Input: dimensioned drawing with shaded views. Units: mm. Origin: part minimum x, y, z. Coordinates: 2 decimals unless noted, no trailing zeros. Order: outer loops, then holes, each group sorted by start corner. A loop starts at its lowest first (then second) coordinate and runs counter-clockwise, first axis right, second up. Notation, with made-up numbers: (-30, 5) - (-18, 5) arc R25 cw to (-18, 41) - close; hole circle Ø9 at (78.5, 4.25). An arc over 180 degrees is marked (long way). Answer as CSV lines item,"result". Start each with the question number.
Item 1: Material intervals for line 1 along X through (y, z) = (8.5, 15.5); line 2 along X through (y, z) = (4.25, 13.5); line 3 along Z through (x, y) = (123.5, 12.75), sorted ascending.
Item 2: Draft query along X for the marked faces 1, 2 and 3. Return one class per face: +X half, -X half, draft (parallel to the pull), parting line (faces both ways), or undercut.
Item 3: Section A-A (y = 4.75). Output: boundary loops of the cut face in (x, z).
Item 4: Section C-C (z = 144.5). Output: boundary loops of the cut face in (x, y), and give its area (3 significant figures).
Item 5: First-contact query: pin 1 (2 mm diameter, centred on y = 3.5, z = 140, fed in from -X); pin 2 (8 mm diameter, centred on y = 6.5, z = 134.5, fed in from -X); pin 3 (8 mm diameter, centred on x = 103, y = 12.5, fed in from +Z). Flat tips, straight axial feed; report the tip coordinate or a pass-through.
Item 6: Section B-B (x = 76.2). Output: boundary loops of the cut face in (y, z).
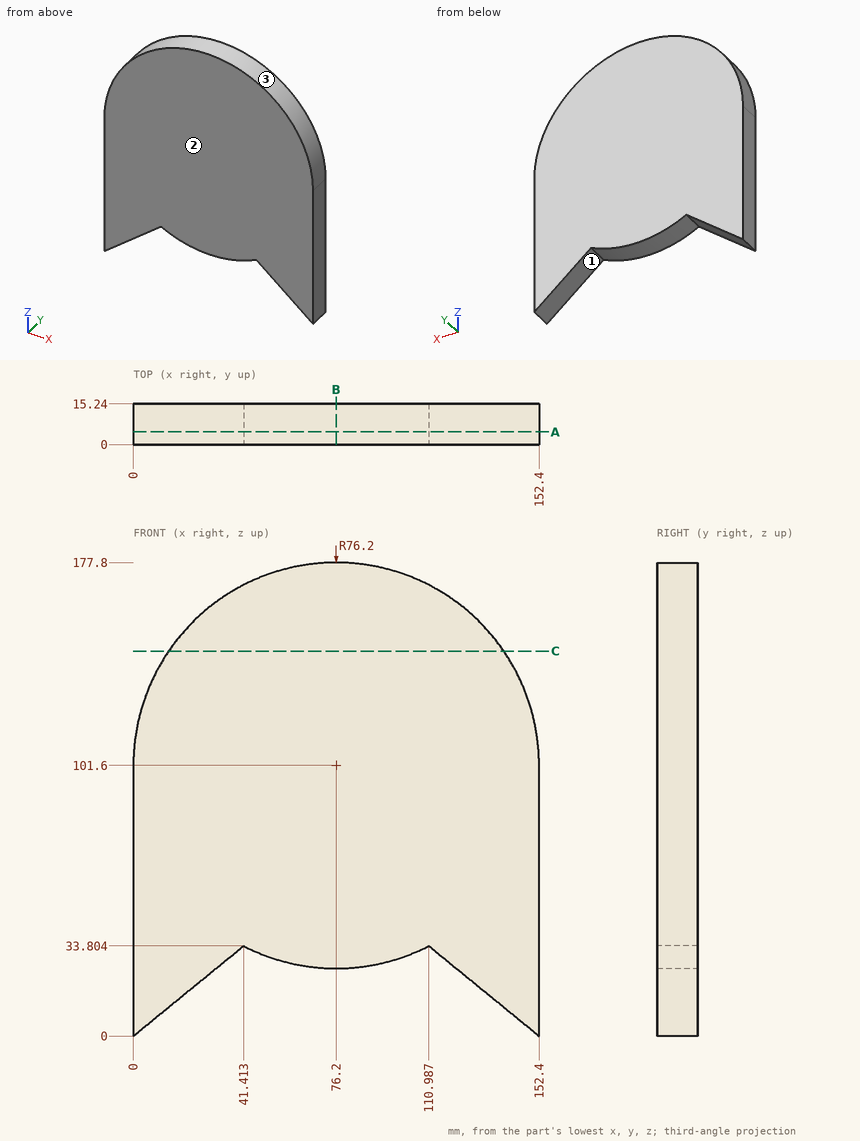
Determined:
1,line 1,"x = 0 to 18.99, 133.41 to 152.4"
1,line 2,"x = 0 to 16.54, 135.86 to 152.4"
1,line 3,"z = 23.59 to 161.34"
2,face 1,"undercut"
2,face 2,"draft"
2,face 3,"parting line"
3,outline,"(0, 0) - (41.41, 33.8) arc R76.2 ccw to (110.99, 33.8) - (152.4, 0) - (152.4, 101.6) arc R76.2 ccw to (0, 101.6) - close"
4,outline,"(13.22, 0) - (139.18, 0) - (139.18, 15.24) - (13.22, 15.24) - close"
4,area,"1,920 mm^2"
5,pin 1,"stops at x = 9.81"
5,pin 2,"stops at x = 5.69"
5,pin 3,"stops at z = 174.31"
6,outline,"(0, 25.4) - (15.24, 25.4) - (15.24, 177.8) - (0, 177.8) - close"
